Input: part model. Units: mm. Frame: model coordinates. A direction names the side the tool comes from. Round coordinates to 2 decimals unless told otherwise and drop trailing zeros. Loops run counter-clockwise (first coordinate to the right, second up) from the corner with the lowest first, then second, coordinate; pieces in that order, holes last. Notation, with made-up numbers: (75.5, 67.5) -> (112.5, 67.5) arc R21 ccw to (112.5, 104.5) -> close; hole circle Ø3 at (75.5, 48). An arc over 180 degrees is marked (long way). One line per question, with ' | ' between items. Start each with the question number.
Q1. Access query for faces 1 (the face through (-165, 152, 1)), 2 (the face through (155, 50, 0)), 3 (the face through (145, 142, 1)). Directions: +Z, -Z, +X, -X, +Y, -Y. A direction counts if a zero-diameter tool reaches every point of the face in a straight line with its end or side. Return the directions, or none.
Q2. Material intervals for L1, parallel to X at y = 288, z = 0; L2, parallel to X at y = 207.5, z = 30; L3, parallel to Z at x = 155, y = 18, sorted ascending.
Q3. Cut plane A-A on y = 41. Return loops of the section in (x, z).
Q4. Mould query, pull axis Z, two halves, no side actions, for faces 4 (the face through (-155, 50, 0)), 5 (the face through (-25, 284, -50)), 6 (the face through (-145, 138, 1)). Classes: pulls with the +Z half, pulls with the -Z half, needs draft (parallel to the pull), parting line crosses it, or undercut.
Q5. Cut plane C-C on z = 36.5. Return loops of the section in (x, y).
Q6. Contact query for flat-ended pins moving along their axis: P1, Ø6, axis at x = -67, z = 19.5, coming from the -Y side; P2, Ø5, axis at x = 155, z = 0, coming from the -Y side; P3, Ø5.5, axis at x = -57, z = 0, coming from the +Y side. Output: stop coordinate, or through.
Q7. Cut plane B-B on y = 136. Return loops of the section in (x, z), and give its area (3 significant figures).
Q8. Cut plane D-D on x = 124. Return loops of the section in (y, z), and give its area (3 significant figures).
from build123d import *

# Parameters (mm, degrees)
BOSS_EXTRUDE1_DEPTH     = 50
SKETCH2_R               = 4
CUT_EXTRUDE1_DEPTH      = 50
CUT_EXTRUDE2_DEPTH      = 347.013005536
CUT_EXTRUDE2_DEPTH_BACK = 347.013005536
SKETCH3_R               = 3


with BuildPart() as part:
    # Sketch1 → Boss-Extrude1 (new, symmetric)
    with BuildSketch(Plane.XY):
        Polygon((-165, 0), (-145, 0), (-145, 280), (145, 280), (145, 0), (165, 0), (165, 300), (-165, 300), align=None)
    extrude(amount=BOSS_EXTRUDE1_DEPTH, both=True)

    # Sketch2 → Cut-Extrude1 (cut)
    with BuildSketch(Plane.XZ):
        with Locations((-155, 0)):
            Circle(SKETCH2_R)
        with Locations(Location((155, 0, 0), (0, 0, 180))):
            Circle(SKETCH2_R)
    extrude(amount=-CUT_EXTRUDE1_DEPTH, mode=Mode.SUBTRACT)

    # Sketch3 → Cut-Extrude2 (cut, two sides: drawn at the far end of the back side and taken through both)
    with BuildSketch(Plane(origin=(0, 300, 0), x_dir=(1, 0, 0), z_dir=(0, 1, 0)).offset(-CUT_EXTRUDE2_DEPTH_BACK)):
        with Locations(Location((-57, 0, 0), (0, 0, 270))):
            Circle(SKETCH3_R)
        with Locations(Location((57, 0, 0), (0, 0, 270))):
            Circle(SKETCH3_R)
    extrude(amount=CUT_EXTRUDE2_DEPTH + CUT_EXTRUDE2_DEPTH_BACK, mode=Mode.SUBTRACT)


solid = part.part
Results:
1) face 1: +Z, -Z, -X, +Y, -Y | face 2: -Y | face 3: +Z, -Z, -Y
2) L1: -165 to -60, -54 to 54, 60 to 165 | L2: -165 to -145, 145 to 165 | L3: -50 to -4, 4 to 50
3) outline: (-165, -50) -> (-145, -50) -> (-145, 50) -> (-165, 50) -> close; (145, -50) -> (165, -50) -> (165, 50) -> (145, 50) -> close; hole circle Ø8 at (-155, 0); hole circle Ø8 at (155, 0)
4) face 4: undercut | face 5: pulls with the -Z half | face 6: needs draft
5) outline: (-165, 0) -> (-145, 0) -> (-145, 280) -> (145, 280) -> (145, 0) -> (165, 0) -> (165, 300) -> (-165, 300) -> close
6) P1: y = 280 | P2: y = 50 | P3: through
7) outline: (-165, -50) -> (-145, -50) -> (-145, 50) -> (-165, 50) -> close; (145, -50) -> (165, -50) -> (165, 50) -> (145, 50) -> close | area: 4,000 mm^2
8) outline: (280, -50) -> (300, -50) -> (300, 50) -> (280, 50) -> close | area: 2,000 mm^2
